The drawing under review shows one solid part. Ordinate dimensions are in mm from its lowest x, y, z. Coordinates: 2 decimals unless noted, no trailing zeros. Write each loop counter-clockwise with the first axis right and the second up, starting at its lowest first coordinate (ties: lowest second). Pieces come first, ordered by that corner, then holes.
1) To check wall thickness, follow line 1 along Y through (x, z) = (378, 1.5); line 2 along X through (y, z) = (593.5, 6). State the ranges of each line that lie inside material, in increasing order.
2) We need section B-B on y = 63. Write out the cut boundary in (x, z).
3) Insertion check: P1, Ø3.5, axis at y = 39, z = 3.5, coming from the -X side; P2, Ø5.5, axis at y = 630.5, z = 3.5, coming from the +X side; P3, Ø3.5, axis at x = 12, z = 4, coming from the +Y side. Each pin has a flat end and moves straight along its axis. Give the tip position at first contact, or say it passes through.
4) We need section A-A on z = 1.75. Write out the cut boundary in (x, y).
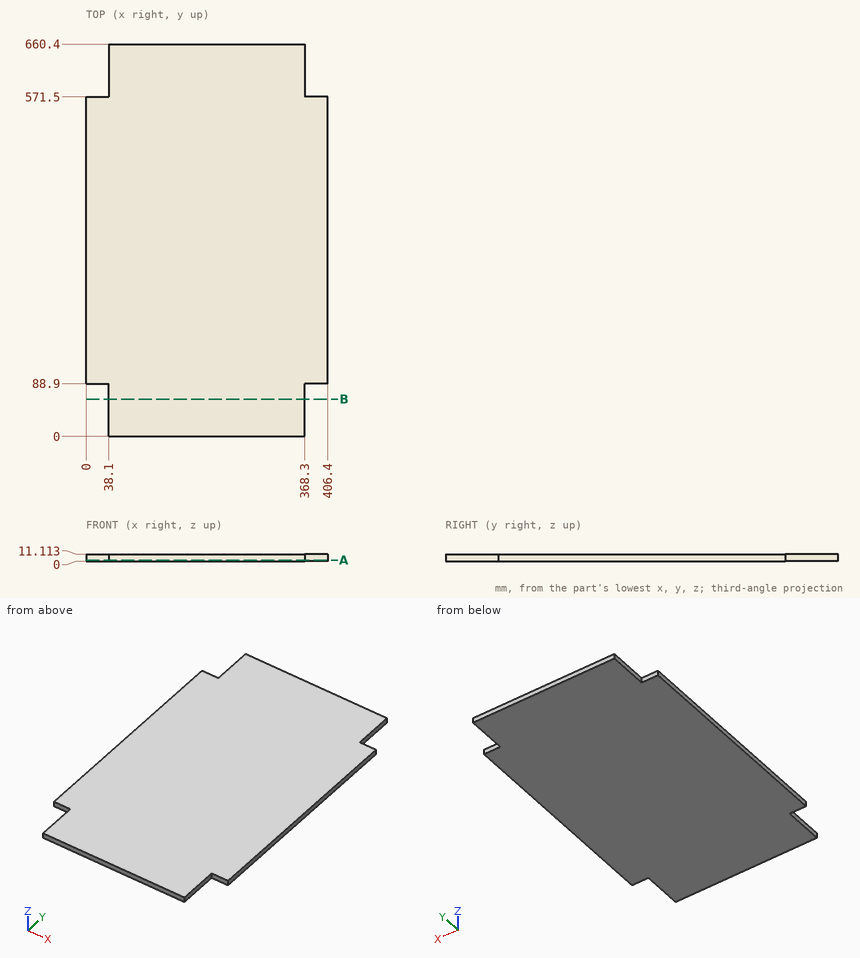
Result:
1. line 1: y = 88.9 to 571.5
1. line 2: x = 38.1 to 368.3
2. outline: (38.1, 0) - (368.3, 0) - (368.3, 11.11) - (38.1, 11.11) - close
3. P1: stops at x = 38.1
3. P2: stops at x = 368.3
3. P3: stops at y = 571.5
4. outline: (0, 88.9) - (38.1, 88.9) - (38.1, 0) - (368.3, 0) - (368.3, 88.9) - (406.4, 88.9) - (406.4, 571.5) - (368.3, 571.5) - (368.3, 660.4) - (38.1, 660.4) - (38.1, 571.5) - (0, 571.5) - close
